from build123d import *

# Parameters (mm, degrees)
SKETCH1_W           = 20
SKETCH1_H           = 9
BOSS_EXTRUDE1_DEPTH = 8
SKETCH2_W           = 8
SKETCH2_H           = 9
BOSS_EXTRUDE2_DEPTH = 10
FILLET1_R           = 3
FILLET3_R           = 1.5


with BuildPart() as part:
    # Sketch1 → Boss-Extrude1 (new body)
    with BuildSketch(Plane(origin=(0, 0, 0), x_dir=(1, 0, 0), z_dir=(0, 1, 0))):
        Rectangle(SKETCH1_W, SKETCH1_H)
        with BuildLine():
            Line((-5.5, 2.5), (-2.5, 2.5))
            ThreePointArc((-2.5, 2.5), (0, 0), (-2.5, -2.5))
            Line((-2.5, -2.5), (-5.5, -2.5))
            ThreePointArc((-5.5, -2.5), (-8, 0), (-5.5, 2.5))
        make_face(mode=Mode.SUBTRACT)
    extrude(amount=BOSS_EXTRUDE1_DEPTH)

    # Sketch2 → Boss-Extrude2 (add)
    with BuildSketch(Plane(origin=(0, 8, 0), x_dir=(1, 0, 0), z_dir=(0, 1, 0))):
        with Locations((6, 0)):
            Rectangle(SKETCH2_W, SKETCH2_H)
    extrude(amount=BOSS_EXTRUDE2_DEPTH)

    # Fillet1
    fillet1_edges = [part.edges().sort_by_distance(p)[0] for p in [
        (-10, 4, 4.5),
        (-10, 4, -4.5),
    ]]
    fillet(fillet1_edges, radius=FILLET1_R)

    # Fillet3
    fillet3_edges = [part.edges().sort_by_distance(p)[0] for p in [
        (2, 13, -4.5),
        (2, 13, 4.5),
        (10, 18, 0),
        (6, 18, -4.5),
        (2, 18, 0),
        (6, 18, 4.5),
        (10, 9, 4.5),
        (10, 9, -4.5),
    ]]
    fillet(fillet3_edges, radius=FILLET3_R)


solid = part.part
The model under review builds one solid part; all positions refer to its coordinate system, in mm. A direction names the side the tool comes from. Round coordinates to 2 decimals unless told otherwise and drop trailing zeros. Loops run counter-clockwise (first coordinate to the right, second up) from the corner with the lowest first, then second, coordinate; pieces in that order, holes last. Notation, with made-up numbers: M 75,5 L 123,5 A26 cw 123,36 Z; hole C -40,59 d1. An arc over 180 degrees is marked long. Answer as a JSON object with one key per item and string values.
Item 1: The part is to be moulded in two halves that separate along Z. For faces 1 (the face through (2.45, 12.31, 4.07)), 2 (the face through (10, 8, 0)), 3 (the face through (-4, 4, -2.5)), say which applies: +Z half, -Z half, draft (parallel to the pull), parting line (faces both ways), or undercut.
Check sheet entries:
{"face 1": "+Z half", "face 2": "draft", "face 3": "undercut"}
Item 2: We need section A-A, the plane x = -4. State the section outline as (y, z) points, and give its area (3 significant figures).
Check sheet entries:
{"outline": "M 0,-4.5 L 8,-4.5 L 8,-2.5 L 0,-2.5 Z; M 0,2.5 L 8,2.5 L 8,4.5 L 0,4.5 Z", "area": "32.0 mm2"}
Item 3: We need section D-D, the plane y = 2.25. State the section outline as (x, z) points.
Check sheet entries:
{"outline": "M -10,-1.5 A3 ccw -7,-4.5 L 8.5,-4.5 A1.5 ccw 10,-3 L 10,3 A1.5 ccw 8.5,4.5 L -7,4.5 A3 ccw -10,1.5 Z; hole M -5.5,-2.5 L -2.5,-2.5 A2.5 ccw -2.5,2.5 L -5.5,2.5 A2.5 ccw Z"}
Item 4: We need section C-C, the plane y = 15. State the section outline as (x, z) points.
Check sheet entries:
{"outline": "M 2,-3 A1.5 ccw 3.5,-4.5 L 8.5,-4.5 A1.5 ccw 10,-3 L 10,3 A1.5 ccw 8.5,4.5 L 3.5,4.5 A1.5 ccw 2,3 Z"}
Item 5: Clearance check with flat-ended pins moving along their axes: P1, Ø1, axis at x = 1, y = 10.5, coming from the -Z side; P2, Ø1.5, axis at x = -4.5, z = -2, coming from the -Y side; P3, Ø3, axis at y = 11, z = 1, coming from the -X side. State where each tip first meets the part, or that it passes through.
Check sheet entries:
{"P1": "through", "P2": "y = 0", "P3": "x = 2"}
Item 6: We need section B-B, the plane z = 0. State the section outline as (x, y) points.
Check sheet entries:
{"outline": "M -10,0 L -8,0 L -8,8 L -10,8 Z; M 0,0 L 10,0 L 10,16.5 A1.5 ccw 8.5,18 L 3.5,18 A1.5 ccw 2,16.5 L 2,8 L 0,8 Z"}
Item 7: For line 1 along Z through (x, y) = (-5.5, 3.5); line 2 along Y through (x, z) = (-5.5, -3.75); line 3 along X through (y, z) = (12, 1.75), list the stretches that pass through material, from the lowest coordinate up.
Check sheet entries:
{"line 1": "-4.5 to -2.5, 2.5 to 4.5", "line 2": "0 to 8", "line 3": "2 to 10"}
Item 8: Tool access review of faces 4 (the face through (0, 4, 0)), 5 (the face through (2.45, 12.31, -4.07)), 6 (the face through (2, 12, 0)): name each direction out of +Z, -Z, +X, -X, +Y, -Y from which nothing blocks a thin tool from reaching the whole face with its end or side.
Check sheet entries:
{"face 4": "+Y, -Y", "face 5": "-Z, -X, +Y", "face 6": "+Z, -Z, -X, +Y"}
